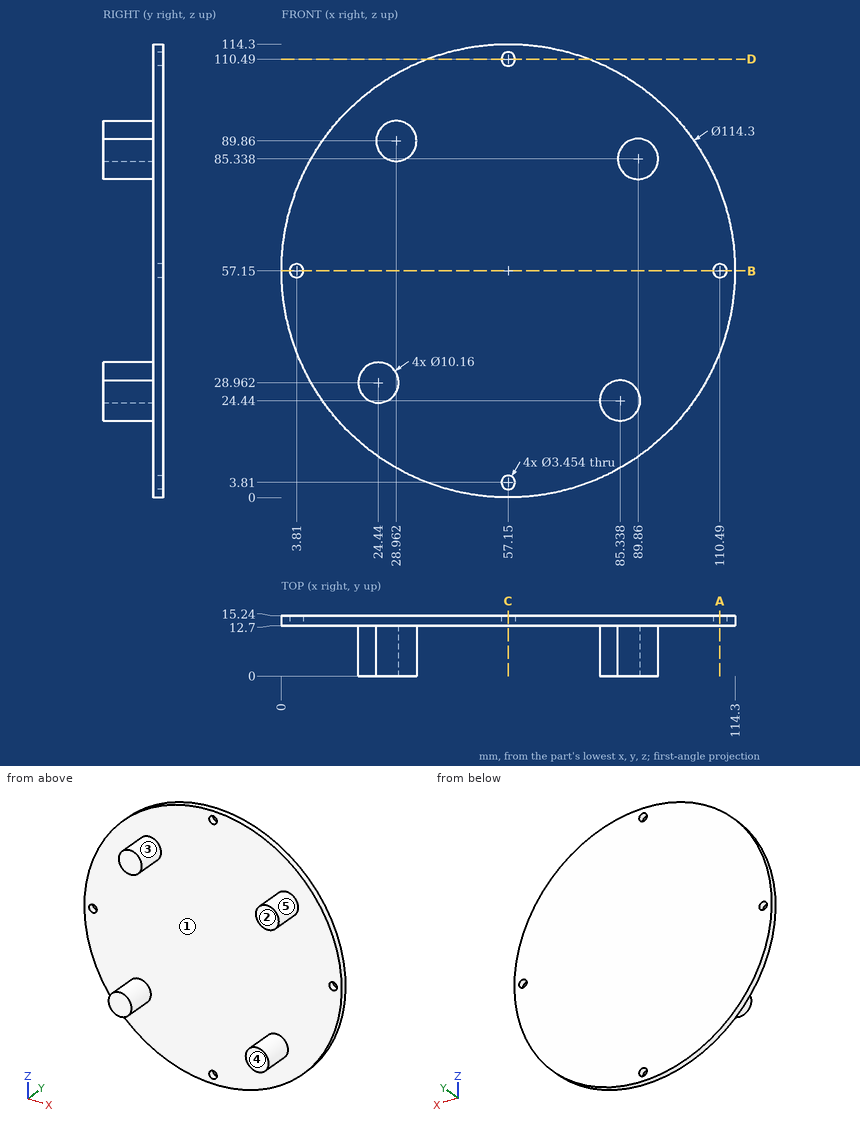
Drawing for the job (mm, zero at the part's lowest x, y, z). A direction names the side the tool comes from. Give positions to 0.01 mm unless a question says otherwise; leave off trailing zeros. Write each loop counter-clockwise with the first axis right and the second up, starting at its lowest first coordinate (ties: lowest second). Pieces come first, ordered by that corner, then holes. Notation, with made-up numbers: (78, 12.5) -> (131, 12.5) arc R17 cw to (131, 35.5) -> close; hole circle Ø3 at (49.5, 81). An arc over 180 degrees is marked (long way). Put each result on its own line as item: value. Start each with the question number.
Item 1: Pin check, flat tips, straight feed: pin 1 Ø2 at (x, y) = (62, 12) entering from -Z; pin 2 Ø5 at (y, z) = (8, 93) entering from -X; pin 3 Ø4 at (x, z) = (57.15, 3.81) entering from -Y. Stop position of each tip, or through.
Item 2: Cut at B-B (z = 57.15). List the corners of the cut face in (x, y).
Item 3: Wall check: L1, parallel to Y at x = 88, z = 38; L2, parallel to X at y = 8.25, z = 25 (1 decimal); L3, parallel to Z at x = 92, y = 5.5 (1 decimal). Give the ranges that are in metal, low to high. Write a range as [from, to].
Item 4: Cut at A-A (x = 110.49). List the corners of the cut face in (y, z).
Item 5: Cut at C-C (x = 57.15). List the corners of the cut face in (y, z), then the cut area to 3 significant figures.
Item 6: Which spindle directions (+Z, -Z, +X, -X, +Y, -Y) get a long thin tool onto all of the face, cutting with end or side? Do the marked faces 1 and 2. Say none if no direction does.
Item 7: Pull direction X, two halves, no side cores. Call the marked faces 3, 4 and 5: pulls with the +X half, pulls with the -X half, needs draft (parallel to the pull), parting line crosses it, or undercut.
Item 8: Cut at D-D (z = 110.49). List the corners of the cut face in (x, y).
Answer list:
1. pin 1: stops at z = 0.15
1. pin 2: stops at x = 23.92
1. pin 3: stops at y = 12.7
2. outline: (0, 12.7) -> (2.08, 12.7) -> (2.08, 15.24) -> (0, 15.24) -> close; (5.54, 12.7) -> (108.76, 12.7) -> (108.76, 15.24) -> (5.54, 15.24) -> close; (112.22, 12.7) -> (114.3, 12.7) -> (114.3, 15.24) -> (112.22, 15.24) -> close
3. L1: y = [12.7, 15.24]
3. L2: x = [21.3, 27.6], [80.3, 90.4]
3. L3: z = [80.7, 89.9]
4. outline: (12.7, 36.63) -> (15.24, 36.63) -> (15.24, 55.42) -> (12.7, 55.42) -> close; (12.7, 58.88) -> (15.24, 58.88) -> (15.24, 77.67) -> (12.7, 77.67) -> close
5. outline: (12.7, 0) -> (15.24, 0) -> (15.24, 2.08) -> (12.7, 2.08) -> close; (12.7, 5.54) -> (15.24, 5.54) -> (15.24, 108.76) -> (12.7, 108.76) -> close; (12.7, 112.22) -> (15.24, 112.22) -> (15.24, 114.3) -> (12.7, 114.3) -> close
5. area: 273 mm2
6. face 1: -Y
6. face 2: +Z, -Z, +X, -X, -Y
7. face 3: undercut
7. face 4: needs draft
7. face 5: undercut
8. outline: (36.63, 12.7) -> (55.42, 12.7) -> (55.42, 15.24) -> (36.63, 15.24) -> close; (58.88, 12.7) -> (77.67, 12.7) -> (77.67, 15.24) -> (58.88, 15.24) -> close
